Autodesk Inventor part; units mm, degrees
ref_plane "YZ Plane" through (0, 0, 0) normal (1, 0, 0) x (0, 1, 0)
ref_plane "XZ Plane" through (0, 0, 0) normal (0, 1, 0) x (-1, 0, 0)
ref_plane "XY Plane" through (0, 0, 0) normal (0, 0, 1) x (1, 0, 0)
sketch "Sketch1" plane through (0, 0, 0) normal (0, 0, 1) x (1, 0, 0)
  circle A0 centre (0, 0) radius 7.45
  circle A1 centre (0, 0) radius 4
  dimension "d0" = 14.9
  dimension "d3" = 8
extrude "Extrusion2" add sketch "Sketch1" along normal blind 20
fillet "Fillet1" radius 0.5 3 edges at (-7.45, 0, 0) (-7.45, 0, 20) (-4, 0, 20)
sketch "Sketch2" plane through (0, 0, 0) normal (0, 0, -1) x (-1, 0, 0)
  circle A0 centre (0, 0) radius 4
  circle A1 centre (0, 0) radius 6.95
  circle A2 centre (0, 0) radius 4
extrude "Extrusion3" add sketch "Sketch2" against normal blind 4.5 contours A0
properties part number "V5 Z Spacer"
Build history of the part. All positions in model axes, mm. A direction names the side the tool comes from. Round coordinates to 2 decimals unless told otherwise and drop trailing zeros. Loops run counter-clockwise (first coordinate to the right, second up) from the corner with the lowest first, then second, coordinate; pieces in that order, holes last. Notation, with made-up numbers: (28, -21) -> (58, -21) arc R34 cw to (58, 16) -> close; hole circle Ø5 at (33.5, 7). An arc over 180 degrees is marked (long way). Answer in a Markdown table with one row per item.
Item 1: Pin check, flat tips, straight feed: pin 1 (1 mm diameter, centred on x = -1, y = -1.5, fed in from -Z); pin 2 (5 mm diameter, centred on x = 3, z = 4, fed in from +Y); pin 3 (4 mm diameter, centred on y = -6, z = 11.5, fed in from -X); pin 4 (2.5 mm diameter, centred on x = 0, y = 0, fed in from +Z). Stop position of each tip, or through.
Answers below:
| item | result |
|---|---|
| pin 1 | stops at z = 0 |
| pin 2 | stops at y = 7.43 |
| pin 3 | stops at x = -6.29 |
| pin 4 | stops at z = 4.5 |
Item 2: Which spindle directions (+Z, -Z, +X, -X, +Y, -Y) get a long thin tool onto all of the face, cutting with end or side? Do faces 4 (the flat face through (0, 0, 0)), 5 (the cylindrical face through (-0.867, 3.905, 11.895)). Say none if no direction does.
Answers below:
| item | result |
|---|---|
| face 4 | -Z, +X, -X, +Y, -Y |
| face 5 | +Z |
Item 3: Mould opens along Y. For faces 1 (the flat face through (0, 0, 4.5)), 2 (the flat face through (5, 0, 20)), 3 (the cylindrical face through (7.106, -2.238, 9.867)) say: +Y half, -Y half, draft (parallel to the pull), parting line (faces both ways), or undercut.
Answers below:
| item | result |
|---|---|
| face 1 | undercut |
| face 2 | draft |
| face 3 | parting line |
Item 4: Saw through at D-D (z = 2). Write the cut outline in (x, y), and give its area (3 significant figures).
Answers below:
| item | result |
|---|---|
| outline | circle Ø14.9 at (0, 0) |
| area | 174 mm² |
Item 5: Drill centre lines: L1, parallel to Y at x = 0, z = 9.5; L2, parallel to Z at x = -2, y = 2.25; L3, parallel to X at y = -2.5, z = 17. Where is each one in solid material? Low to high. Write a range as [from, to].
Answers below:
| item | result |
|---|---|
| L1 | y = [-7.45, -4], [4, 7.45] |
| L2 | z = [0, 4.5] |
| L3 | x = [-7.02, -3.12], [3.12, 7.02] |
Item 6: Saw through at C-C (z = 12.75). Write the cut outline in (x, y).
Answers below:
| item | result |
|---|---|
| outline | circle Ø14.9 at (0, 0); hole circle Ø8 at (0, 0) |
Item 7: Saw through at A-A (y = 0). Write the cut outline in (x, z), and give its area (3 significant figures).
Answers below:
| item | result |
|---|---|
| outline | (-7.45, 0.5) arc R0.5 ccw to (-6.95, 0) -> (6.95, 0) arc R0.5 ccw to (7.45, 0.5) -> (7.45, 19.5) arc R0.5 ccw to (6.95, 20) -> (4.5, 20) arc R0.5 ccw to (4, 19.5) -> (4, 4.5) -> (-4, 4.5) -> (-4, 19.5) arc R0.5 ccw to (-4.5, 20) -> (-6.95, 20) arc R0.5 ccw to (-7.45, 19.5) -> close |
| area | 174 mm² |
